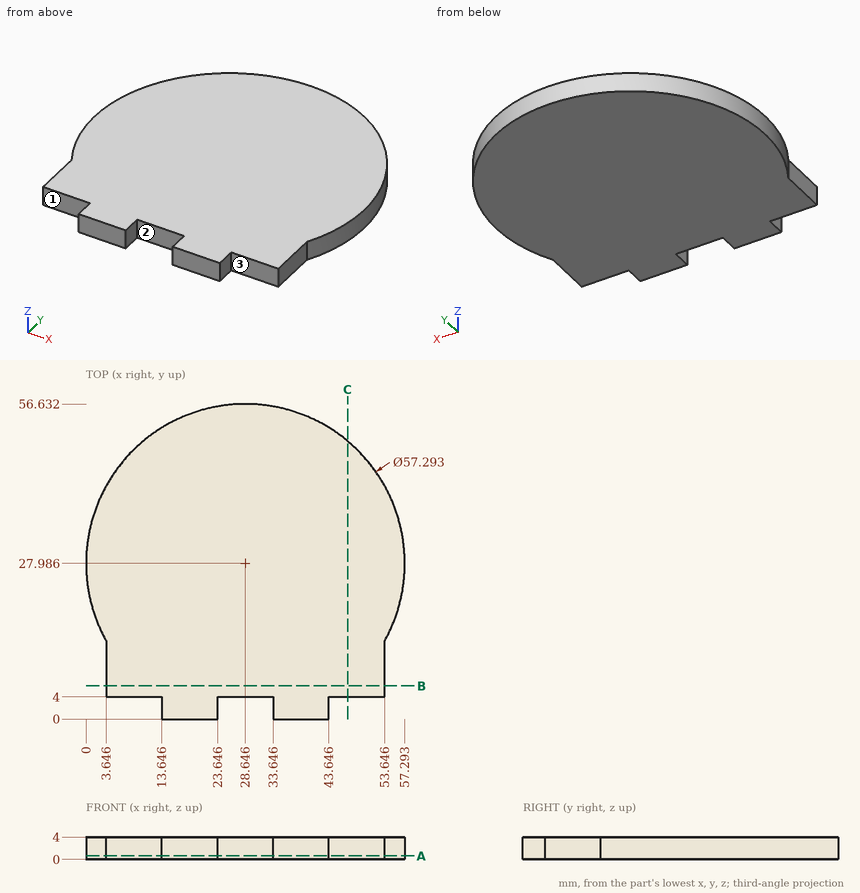
Job drawing, mm, ordinate dimensions from the low corner. One solid piece. A direction names the side the tool comes from. Coordinates: 2 decimals unless noted, no trailing zeros. Loops run counter-clockwise (first coordinate to the right, second up) from the corner with the lowest first, then second, coordinate; pieces in that order, holes last. Notation, with made-up numbers: (35, 10) - (53, 10) arc R20 ccw to (53, 38) - close; hole circle Ø9 at (18, 74.5). An arc over 180 degrees is marked (long way). Answer as a JSON object with one key per item and string values. Group by question number.
(1) Tool access for the marked faces 1, 2 and 3: list every direction of +Z, -Z, +X, -X, +Y, -Y with a clear straight run to the whole face (end or side of a thin tool).
(2) Probe line 1 along X through (y, z) = (2.5, 2.6); line 2 along X through (y, z) = (7.5, 1.7); line 3 along Y through (x, z) = (37.5, 1). List the from-to ranges inside material, lowest first.
(3) Cut at C-C (x = 47). Give the cut face in (y, z).
(4) Flat gauge pins, fed straight in: pin 1 (2 mm diameter, centred on y = 2.5, z = 2, fed in from -X); pin 2 (1.2 mm diameter, centred on x = 30, z = 2, fed in from -Y); pin 3 (1.2 mm diameter, centred on y = 2, z = 2, fed in from +X). Where does each tip first touch, or does it go through?
(5) Cut at A-A (z = 0.65). Give the cut face in (x, y), then the cut area to 3 significant figures.
(6) Cut at B-B (y = 6). Give the cut face in (x, z).
Geometry says:
{
 "1": {"face 1": "+Z, -Z, -X, -Y", "face 2": "+Z, -Z, -Y", "face 3": "+Z, -Z, +X, -Y"},
 "2": {"line 1": "x = 13.65 to 23.65, 33.65 to 43.65", "line 2": "x = 3.65 to 53.65", "line 3": "y = 0 to 55.23"},
 "3": {"outline": "(4, 0) - (49.98, 0) - (49.98, 4) - (4, 4) - close"},
 "4": {"pin 1": "stops at x = 13.65", "pin 2": "stops at y = 4", "pin 3": "stops at x = 43.65"},
 "5": {"outline": "(3.65, 4) - (13.65, 4) - (13.65, 0) - (23.65, 0) - (23.65, 4) - (33.65, 4) - (33.65, 0) - (43.65, 0) - (43.65, 4) - (53.65, 4) - (53.65, 14) arc R28.65 ccw (long way) to (3.65, 14) - close", "area": "2,640 mm^2"},
 "6": {"outline": "(3.65, 0) - (53.65, 0) - (53.65, 4) - (3.65, 4) - close"}
}
